Verification items for the finished model (mm, model axes). A direction names the side the tool comes from. Coordinates: 2 decimals unless noted, no trailing zeros. Loops run counter-clockwise (first coordinate to the right, second up) from the corner with the lowest first, then second, coordinate; pieces in that order, holes last. Notation, with made-up numbers: (18, 16) -> (46, 16) arc R19 ccw to (46, 52) -> close; hole circle Ø8 at (-29, 67). An arc over 180 degrees is marked (long way). Answer as a JSON object with one key per item and string values. Group by question number.
Q1. Scan lines: L1, parallel to X at y = 1, z = 0; L2, parallel to Y at x = 41, z = -73.5; L3, parallel to X at y = -61, z = 22. Record each from-to range of solid material in increasing order.
Q2. Cross-section at B-B on z = -31. Record the boundary of the cut face in (x, y), and give its area (3 significant figures).
Q3. Gauge pin test, flat ends, axial feed: pin 1 Ø1 at (x, y) = (57, 1) entering from +Z; pin 2 Ø0.6 at (x, y) = (-51.5, -21.5) entering from -Z; pin 3 Ø10 at (x, y) = (-15.5, -57) entering from +Z. Record the tip position at first contact, or that the pin passes through.
Q4. Release check for a two-part mould opening along Z. For faces 1 (the flat face through (-33.674, 1.014, 49.84)), 2 (the cylindrical face through (42.224, -41.905, 32.033)), 3 (the flat face through (-23.83, 1.01, -49.75)), 4 (the flat face through (-48, -85, 19)) record: released by +Z, released by -Z, zero draft, split by the parting line, or undercut.
Q5. Cross-section at D-D on z = 68. Record the boundary of the cut face in (x, y).
Q6. Cross-section at A-A on y = -67. Record the boundary of the cut face in (x, z), and give its area (3 significant figures).
Q7. Set-up check for faces 5 (the cylindrical face through (-47.224, -41.905, 19.258)), 6 (the flat face through (-26.3, 1, -54.1)), 7 (the flat face through (-3.011, -30.42, -51.747)): record each of +Z, -Z, +X, -X, +Y, -Y from which the full face is reachable in a straight line by a thin tool's end or side.
Q8. Cross-section at C-C on y = -51.5. Record the boundary of the cut face in (x, z), and give its area (3 significant figures).
```python
from build123d import *

# Parameters (mm, degrees)
SKETCH3_R           = 90
BOSS_EXTRUDE3_DEPTH = 2
SKETCH4_R           = 45
CUT_EXTRUDE1_DEPTH  = 2
BOSS_EXTRUDE4_DEPTH = 85
BOSS_EXTRUDE5_DEPTH = 85
CUT_EXTRUDE9_DEPTH  = 10
CIRPATTERN4_COUNT   = 3
CUT_EXTRUDE5_DEPTH  = 60
SKETCH15_W          = 5
SKETCH15_H          = 25
CUT_EXTRUDE10_DEPTH = 88.0000001
CIRPATTERN5_COUNT   = 3
SKETCH16_R          = 46
CUT_EXTRUDE11_DEPTH = 85
BOSS_EXTRUDE6_DEPTH = 2
SKETCH18_W          = 18.5
SKETCH18_H          = 12
CUT_EXTRUDE12_DEPTH = 2


with BuildPart() as part:
    # Sketch3 → Boss-Extrude3 (new body)
    with BuildSketch(Plane(origin=(0, 0, 0), x_dir=(1, 0, 0), z_dir=(0, 1, 0))):
        Circle(SKETCH3_R)
    extrude(amount=BOSS_EXTRUDE3_DEPTH)

    # Sketch4 → Cut-Extrude1 (cut)
    with BuildSketch(Plane.XZ):
        Circle(SKETCH4_R)
    extrude(amount=-CUT_EXTRUDE1_DEPTH, mode=Mode.SUBTRACT)

    # Sketch6 → Boss-Extrude4 (add)
    with BuildSketch(Plane.XZ):
        with BuildLine():
            Line((-46, 0), (-45, 0))
            ThreePointArc((-45, 0), (-41.574578963, 17.220754456), (-31.819805153, 31.819805153))
            Line((-31.819805153, 31.819805153), (-32.526911935, 32.526911935))
            ThreePointArc((-32.526911935, 32.526911935), (-42.498458496, 17.603437889), (-46, 0))
        make_face()
    boss_extrude4 = extrude(amount=BOSS_EXTRUDE4_DEPTH)

    # Sketch6<3> → Boss-Extrude5 (add)
    with BuildSketch(Plane.XZ):
        with BuildLine():
            Line((-53, 0), (-51, 0))
            ThreePointArc((-51, 0), (-47.117856158, 19.516855051), (-36.062445841, 36.062445841))
            Line((-36.062445841, 36.062445841), (-37.476659403, 37.476659403))
            ThreePointArc((-37.476659403, 37.476659403), (-48.965615223, 20.282221915), (-53, 0))
        make_face()
    boss_extrude5 = extrude(amount=BOSS_EXTRUDE5_DEPTH)

    # Sketch14 → Cut-Extrude9 (cut)
    with BuildSketch(Plane(origin=(-38.409902577, 0, 15.909902577), x_dir=(-0.382683432, 0, -0.923879533), z_dir=(0.923879533, 0, -0.382683432))):
        with BuildLine():
            Line((1.5, -75), (1.5, -83))
            ThreePointArc((1.5, -83), (0, -84.5), (-1.5, -83))
            Line((-1.5, -83), (-1.5, -75))
            ThreePointArc((-1.5, -75), (0, -73.5), (1.5, -75))
        make_face()
    cut_extrude9 = extrude(amount=-CUT_EXTRUDE9_DEPTH, mode=Mode.SUBTRACT)

    # CirPattern4: Boss-Extrude4, Boss-Extrude5, Cut-Extrude9 ×3 about axis
    cirpattern4_axis = Axis((0, 0, 0), (0, 1, 0))
    for i in range(1, CIRPATTERN4_COUNT):
        add(boss_extrude4.rotate(cirpattern4_axis, i * 360 / CIRPATTERN4_COUNT))
        add(boss_extrude5.rotate(cirpattern4_axis, i * 360 / CIRPATTERN4_COUNT))
        add(cut_extrude9.rotate(cirpattern4_axis, i * 360 / CIRPATTERN4_COUNT), mode=Mode.SUBTRACT)

    # Sketch11 → Cut-Extrude5 (cut, symmetric)
    with BuildSketch(Plane.XZ):
        Polygon((-6.747570404, -52.479477871), (11.40662685, -48.919264104), (13.715954699, -60.69495962), (-4.438242555, -64.255173387), align=None)
    extrude(amount=CUT_EXTRUDE5_DEPTH, both=True, mode=Mode.SUBTRACT)

    # Sketch15 → Cut-Extrude10 (cut, through all)
    with BuildSketch(Plane(origin=(0, 2, 0), x_dir=(1, 0, 0), z_dir=(0, 1, 0))):
        with Locations((57.5, -4.067185812)):
            Rectangle(SKETCH15_W, SKETCH15_H)
    cut_extrude10 = extrude(amount=-CUT_EXTRUDE10_DEPTH, mode=Mode.SUBTRACT)

    # CirPattern5: Cut-Extrude10 ×3 about axis
    cirpattern5_axis = Axis((0, 0, 0), (0, 1, 0))
    for i in range(1, CIRPATTERN5_COUNT):
        add(cut_extrude10.rotate(cirpattern5_axis, i * 360 / CIRPATTERN5_COUNT), mode=Mode.SUBTRACT)

    # Sketch16 → Cut-Extrude11 (cut)
    with BuildSketch(Plane.XZ.offset(85)):
        Circle(SKETCH16_R)
    extrude(amount=-CUT_EXTRUDE11_DEPTH, mode=Mode.SUBTRACT)

    # Sketch17 → Boss-Extrude6 (add)
    with BuildSketch(Plane(origin=(0, 2, 0), x_dir=(1, 0, 0), z_dir=(0, 1, 0))):
        Polygon((13.715954699, 60.69495962), (-4.438242555, 64.255173387), (-6.747570404, 52.479477871), (11.40662685, 48.919264104), align=None)
    extrude(amount=-BOSS_EXTRUDE6_DEPTH)

    # Sketch18 → Cut-Extrude12 (cut)
    with BuildSketch(Plane(origin=(0, 2, 0), x_dir=(1, 0, 0), z_dir=(0, 1, 0))):
        with Locations((9.25, -56)):
            Rectangle(SKETCH18_W, SKETCH18_H)
    extrude(amount=-CUT_EXTRUDE12_DEPTH, mode=Mode.SUBTRACT)


solid = part.part
```
Computed values:
{
 "1": {"L1": "x = -90 to -45, 45 to 55, 60 to 90", "L2": "y = 0 to 2", "L3": "x = -48.22 to -46.01, 46.01 to 48.22"},
 "2": {"outline": "(-84.49, 0) -> (-32.62, 0) -> (-32.62, 2) -> (-84.49, 2) -> close; (32.62, 0) -> (84.49, 0) -> (84.49, 2) -> (32.62, 2) -> close", "area": "207 mm²"},
 "3": {"pin 1": "stops at z = 70.06", "pin 2": "stops at z = 0", "pin 3": "stops at z = -49.26"},
 "4": {"face 1": "undercut", "face 2": "released by +Z", "face 3": "undercut", "face 4": "zero draft"},
 "5": {"outline": "(-58.96, 0) -> (58.96, 0) -> (58.96, 2) -> (-58.96, 2) -> close"},
 "6": {"outline": "(-53, 0) -> (-51, 0) arc R51 cw to (-36.06, 36.06) -> (-37.48, 37.48) arc R53 ccw to start; (-13.72, -51.19) arc R53 ccw to (26.5, -45.9) -> (25.5, -44.17) arc R51 cw to (-13.2, -49.26) -> close; (25.5, 44.17) arc R51 cw to (49.26, 13.2) -> (51.19, 13.72) arc R53 ccw to (26.5, 45.9) -> close", "area": "245 mm²"},
 "7": {"face 5": "-Z, -Y", "face 6": "+Y, -Y", "face 7": "-Z"},
 "8": {"outline": "(-53, 0) -> (-51, 0) arc R51 cw to (-36.06, 36.06) -> (-37.48, 37.48) arc R53 ccw to start; (-13.72, -51.19) arc R53 ccw to (-6.73, -52.57) -> (-6.75, -52.48) -> (0.83, -50.99) arc R51 cw to (-13.2, -49.26) -> close; (11.55, -49.67) -> (11.94, -51.64) arc R53 ccw to (26.5, -45.9) -> (25.5, -44.17) arc R51 cw to start; (25.5, 44.17) arc R51 cw to (49.26, 13.2) -> (51.19, 13.72) arc R53 ccw to (26.5, 45.9) -> close", "area": "214 mm²"}
}
